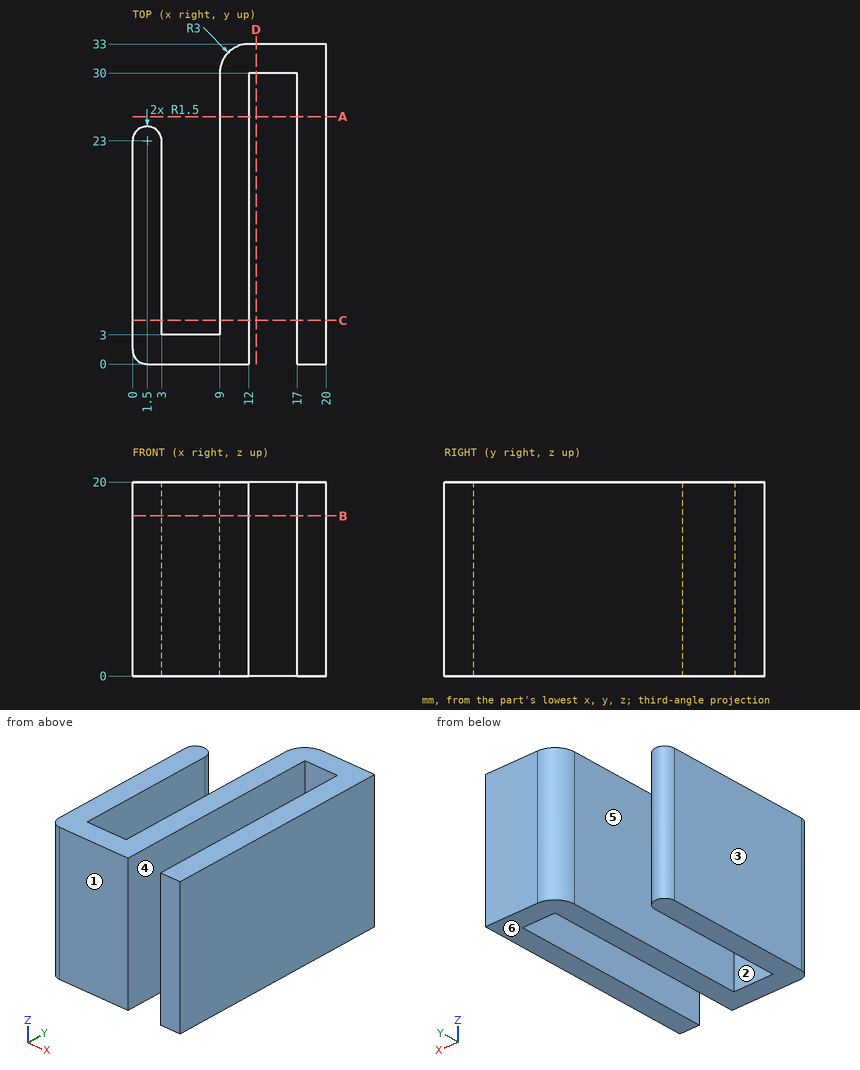
Input: dimensioned drawing with shaded views. Units: mm. Origin: part minimum x, y, z. A direction names the side the tool comes from. Round coordinates to 2 decimals unless told otherwise and drop trailing zeros. Order: outer loops, then holes, each group sorted by start corner. A loop starts at its lowest first (then second) coordinate and runs counter-clockwise, first axis right, second up. Notation, with made-up numbers: (35, -3) - (83, -3) arc R21 ccw to (83, 31) - close; hole circle Ø3 at (16, 47). An arc over 180 degrees is marked (long way). Use CSV: the item, a comma, the result in double quotes. Start each with the question number.
Q1. Access query for the marked faces 4, 5 and 6. Directions: +Z, -Z, +X, -X, +Y, -Y. A direction counts if a zero-diameter tool reaches every point of the face in a straight line with its end or side. Return the directions, or none.
Q2. Section query C-C (y = 4.5). Return loops of the section in (x, z), and give its area (3 significant figures).
Q3. Material intervals for line 1 along X through (y, z) = (6, 6.75); line 2 along X through (y, z) = (28.5, 2); line 3 along Y through (x, z) = (7.25, 9.5), sorted ascending. Write a range as from..to.
Q4. First-contact query: pin 1 (10 mm diameter, centred on x = 15, y = 24.5, fed in from +Z); pin 2 (3 mm diameter, centred on x = 5, z = 14, fed in from +Y); pin 3 (2.5 mm diameter, centred on x = 13.5, z = 5.5, fed in from -Y); pin 4 (5 mm diameter, centred on y = 26, z = 17, fed in from -X). Flat tips, straight axial feed; report the tip coordinate or a pass-through.
Q5. Section query B-B (z = 16.5). Return loops of the section in (x, y), and give its area (3 significant figures).
Q6. Section query D-D (x = 12.75). Return loops of the section in (y, z).
Q7. Mould query, pull axis X, two halves, no side actions, for the marked faces 1, 2 and 3. Classes: +X half, -X half, draft (parallel to the pull), parting line (faces both ways), or undercut.
Q8. Section query A-A (y = 25.5). Return loops of the section in (x, z), and give its area (3 significant figures).
Result set:
1,face 4,"+Z, -Z, -Y"
1,face 5,"+Z, -Z, +Y"
1,face 6,"-Z, +X, -X, +Y, -Y"
2,outline,"(0, 0) - (3, 0) - (3, 20) - (0, 20) - close; (9, 0) - (12, 0) - (12, 20) - (9, 20) - close; (17, 0) - (20, 0) - (20, 20) - (17, 20) - close"
2,area,"180 mm2"
3,line 1,"x = 0..3, 9..12, 17..20"
3,line 2,"x = 9..12, 17..20"
3,line 3,"y = 0..3"
4,pin 1,"stops at z = 20"
4,pin 2,"stops at y = 3"
4,pin 3,"stops at y = 30"
4,pin 4,"stops at x = 0.09"
5,outline,"(0, 1.5) arc R1.5 ccw to (1.5, 0) - (12, 0) - (12, 30) - (17, 30) - (17, 0) - (20, 0) - (20, 33) - (12, 33) arc R3 ccw to (9, 30) - (9, 3) - (3, 3) - (3, 23) arc R1.5 ccw to (0, 23) - close"
5,area,"301 mm2"
6,outline,"(30, 0) - (33, 0) - (33, 20) - (30, 20) - close"
7,face 1,"draft"
7,face 2,"undercut"
7,face 3,"-X half"
8,outline,"(9, 0) - (12, 0) - (12, 20) - (9, 20) - close; (17, 0) - (20, 0) - (20, 20) - (17, 20) - close"
8,area,"120 mm2"
